Part model, mm, in its own coordinate system. Give positions to 0.01 mm unless a question says otherwise; leave off trailing zeros. Loops run counter-clockwise (first coordinate to the right, second up) from the corner with the lowest first, then second, coordinate; pieces in that order, holes last. Notation, with made-up numbers: (34.5, 39.5) -> (60.5, 39.5) arc R21 cw to (60.5, 73.5) -> close; hole circle Ø4 at (-29, 3.5). An arc over 180 degrees is marked (long way). One line per question, with ' | ' between items.
```python
from build123d import *

# Parameters (mm, degrees)
F0_W     = 38.1
F0_H     = 38.1
F0_W_2   = 25.4
F0_H_2   = 25.4
F1_DEPTH = 977.9
F2_R     = 12.7
F3_DEPTH = 317.5
F4_R     = 6.35
F5_DEPTH = 76.2
F7_DEPTH = 50.8


with BuildPart() as f1:
    # F0 (on Front) → F1 (new body, symmetric)
    with BuildSketch(Plane.XZ):
        Rectangle(F0_W, F0_H)
        Rectangle(F0_W_2, F0_H_2, mode=Mode.SUBTRACT)
    extrude(amount=F1_DEPTH, both=True)

    # F2 (on Top) → F3 (cut, symmetric)
    with BuildSketch(Plane.XY):
        with Locations((0, -952.5)):
            Circle(F2_R)
        with Locations((0, 952.5)):
            Circle(F2_R)
    extrude(amount=F3_DEPTH, both=True, mode=Mode.SUBTRACT)

    # F4 (on face) → F5 (cut)
    with BuildSketch(Plane.YZ.offset(19.05)):
        with Locations((892.175, 0)):
            Circle(F4_R)
    extrude(amount=-F5_DEPTH, mode=Mode.SUBTRACT)

    # F6 (on face) → F7 (cut)
    with BuildSketch(Plane.YZ.offset(19.05)):
        with BuildLine():
            Line((-854.075, 6.35), (-930.275, 6.35))
            ThreePointArc((-930.275, 6.35), (-936.625, 0), (-930.275, -6.35))
            Line((-930.275, -6.35), (-854.075, -6.35))
            ThreePointArc((-854.075, -6.35), (-847.725, 0), (-854.075, 6.35))
        make_face()
    extrude(amount=-F7_DEPTH, mode=Mode.SUBTRACT)


solid = f1.part
```
1) Saw through at B-B (y = 485). Give the cut face in (x, z), and give its area (3 significant figures).
Found:
outline: (-19.05, -19.05) -> (19.05, -19.05) -> (19.05, 19.05) -> (-19.05, 19.05) -> close; hole (-12.7, -12.7) -> (12.7, -12.7) -> (12.7, 12.7) -> (-12.7, 12.7) -> close | area: 806 mm2
2) Pull direction Y, two halves, no side cores. Call faces 1 (the flat face through (-13, -977.9, 0)), 2 (the flat face through (0, -14, 19.05)), 3 (the flat face through (-13, 977.9, 0)): pulls with the +Y half, pulls with the -Y half, needs draft (parallel to the pull), parting line crosses it, or undercut.
Found:
face 1: pulls with the -Y half | face 2: needs draft | face 3: pulls with the +Y half
3) Saw through at A-A (x = 0). Give the cut face in (y, z), and give its area (3 significant figures).
Found:
outline: (-977.9, -19.05) -> (-965.2, -19.05) -> (-965.2, -12.7) -> (-977.9, -12.7) -> close; (-977.9, 12.7) -> (-965.2, 12.7) -> (-965.2, 19.05) -> (-977.9, 19.05) -> close; (-939.8, -19.05) -> (939.8, -19.05) -> (939.8, -12.7) -> (-939.8, -12.7) -> close; (-939.8, 12.7) -> (939.8, 12.7) -> (939.8, 19.05) -> (-939.8, 19.05) -> close; (965.2, -19.05) -> (977.9, -19.05) -> (977.9, -12.7) -> (965.2, -12.7) -> close; (965.2, 12.7) -> (977.9, 12.7) -> (977.9, 19.05) -> (965.2, 19.05) -> close | area: 24,200 mm2
4) Saw through at C-C (z = 0). Give the cut face in (x, y) (3 decimals).
Found:
outline: (-19.05, -977.9) -> (-12.7, -977.9) -> (-12.7, -936.625) -> (-19.05, -936.625) -> close; (-19.05, -847.725) -> (-12.7, -847.725) -> (-12.7, 885.825) -> (-19.05, 885.825) -> close; (-19.05, 898.525) -> (-12.7, 898.525) -> (-12.7, 977.9) -> (-19.05, 977.9) -> close; (12.7, -977.9) -> (19.05, -977.9) -> (19.05, -936.625) -> (12.7, -936.625) -> close; (12.7, -847.725) -> (19.05, -847.725) -> (19.05, 885.825) -> (12.7, 885.825) -> close; (12.7, 898.525) -> (19.05, 898.525) -> (19.05, 977.9) -> (12.7, 977.9) -> close
5) Drill centre lines: line 1 (Y direction, x = 0, z = 14); line 2 (Y direction, x = -2.5, z = 13); line 3 (Z direction, x = -12, y = 652). Where is each one in solid material? Low to high.
Found:
line 1: -977.9 to -965.2, -939.8 to 939.8, 965.2 to 977.9 | line 2: -977.9 to -964.95, -940.05 to 940.05, 964.95 to 977.9 | line 3: -19.05 to -12.7, 12.7 to 19.05
